Verification items for the finished model (mm, model axes). A direction names the side the tool comes from. Coordinates: 2 decimals unless noted, no trailing zeros. Loops run counter-clockwise (first coordinate to the right, second up) from the corner with the lowest first, then second, coordinate; pieces in that order, holes last. Notation, with made-up numbers: M 30.25,1 L 89.25,1 A24 cw 89.25,36 Z; hole C 73.5,68 d2. An arc over 180 degrees is marked long. Write item = value, one per line. Start each with the question number.
```python
from build123d import *

# Parameters (mm, degrees)
SKETCH_1_W          = 100
SKETCH_1_H          = 100
EXTRUDE_1_DEPTH     = 100
SKETCH_2_W          = 90
SKETCH_2_H          = 75
CUT_EXTRUDE_1_DEPTH = 151
CUT_EXTRUDE_2_REACH = 124.474
SKETCH_3_R          = 7.5
CUT_EXTRUDE_3_REACH = 112.567
SKETCH_4_R          = 1.5
CUT_EXTRUDE_4_DEPTH = 5
SKETCH_6_R          = 1.5
CUT_EXTRUDE_5_DEPTH = 5


with BuildPart() as part:
    # 草圖1 → 填料-伸長1 (new body)
    with BuildSketch(Plane.XY):
        Rectangle(SKETCH_1_W, SKETCH_1_H)
    extrude(amount=EXTRUDE_1_DEPTH)

    # 草圖2 → 除料-伸長1 (cut, through all)
    with BuildSketch(Plane.XZ.offset(50)):
        with Locations((0, 47.5)):
            Rectangle(SKETCH_2_W, SKETCH_2_H)
    extrude(amount=-CUT_EXTRUDE_1_DEPTH, mode=Mode.SUBTRACT)

    # 草圖3 → 除料-伸長2 (cut, up to next)
    with BuildSketch(Plane(origin=(0, 0, 0), x_dir=(-1, 0, 0), z_dir=(0, 0, -1)), mode=Mode.PRIVATE) as cut_extrude_2_sk1:
        Circle(SKETCH_3_R)
    cut_extrude_2_tool1 = extrude(cut_extrude_2_sk1.sketch, amount=-CUT_EXTRUDE_2_REACH, mode=Mode.PRIVATE) & part.part
    add(cut_extrude_2_tool1.solids().sort_by_distance((0, 0, 0))[0], mode=Mode.SUBTRACT)

    # 草圖4 → 除料-伸長3 (cut, up to next)
    with BuildSketch(Plane(origin=(0, 0, 85), x_dir=(-1, 0, 0), z_dir=(0, 0, -1)), mode=Mode.PRIVATE) as cut_extrude_3_sk1:
        with Locations((-32.4, 11.9)):
            Circle(SKETCH_4_R)
    cut_extrude_3_tool1 = extrude(cut_extrude_3_sk1.sketch, amount=-CUT_EXTRUDE_3_REACH, mode=Mode.PRIVATE) & part.part
    # 草圖4 → 除料-伸長3 (cut, up to next)
    with BuildSketch(Plane(origin=(0, 0, 85), x_dir=(-1, 0, 0), z_dir=(0, 0, -1)), mode=Mode.PRIVATE) as cut_extrude_3_sk2:
        with Locations(Location((32.4, 11.9, 0), (0, 0, 180))):
            Circle(SKETCH_4_R)
    cut_extrude_3_tool2 = extrude(cut_extrude_3_sk2.sketch, amount=-CUT_EXTRUDE_3_REACH, mode=Mode.PRIVATE) & part.part
    # 草圖4 → 除料-伸長3 (cut, up to next)
    with BuildSketch(Plane(origin=(0, 0, 85), x_dir=(-1, 0, 0), z_dir=(0, 0, -1)), mode=Mode.PRIVATE) as cut_extrude_3_sk3:
        with Locations((32.4, -11.9)):
            Circle(SKETCH_4_R)
    cut_extrude_3_tool3 = extrude(cut_extrude_3_sk3.sketch, amount=-CUT_EXTRUDE_3_REACH, mode=Mode.PRIVATE) & part.part
    # 草圖4 → 除料-伸長3 (cut, up to next)
    with BuildSketch(Plane(origin=(0, 0, 85), x_dir=(-1, 0, 0), z_dir=(0, 0, -1)), mode=Mode.PRIVATE) as cut_extrude_3_sk4:
        with Locations(Location((-32.4, -11.9, 0), (0, 0, 180))):
            Circle(SKETCH_4_R)
    cut_extrude_3_tool4 = extrude(cut_extrude_3_sk4.sketch, amount=-CUT_EXTRUDE_3_REACH, mode=Mode.PRIVATE) & part.part
    # 草圖4 → 除料-伸長3 (cut, up to next)
    with BuildSketch(Plane(origin=(0, 0, 85), x_dir=(-1, 0, 0), z_dir=(0, 0, -1)), mode=Mode.PRIVATE) as cut_extrude_3_sk5:
        with BuildLine():
            Line((24.9, 24.4), (-24.9, 24.4))
            ThreePointArc((-24.9, 24.4), (-26.314213562, 23.814213562), (-26.9, 22.4))
            Line((-26.9, 22.4), (-26.9, -22.4))
            ThreePointArc((-26.9, -22.4), (-26.314213562, -23.814213562), (-24.9, -24.4))
            Line((-24.9, -24.4), (24.9, -24.4))
            ThreePointArc((24.9, -24.4), (26.314213562, -23.814213562), (26.9, -22.4))
            Line((26.9, -22.4), (26.9, 22.4))
            ThreePointArc((26.9, 22.4), (26.314213562, 23.814213562), (24.9, 24.4))
        make_face()
    cut_extrude_3_tool5 = extrude(cut_extrude_3_sk5.sketch, amount=-CUT_EXTRUDE_3_REACH, mode=Mode.PRIVATE) & part.part
    add(cut_extrude_3_tool1.solids().sort_by_distance((32.4, 11.9, 85))[0], mode=Mode.SUBTRACT)
    add(cut_extrude_3_tool2.solids().sort_by_distance((-32.4, 11.9, 85))[0], mode=Mode.SUBTRACT)
    add(cut_extrude_3_tool3.solids().sort_by_distance((-32.4, -11.9, 85))[0], mode=Mode.SUBTRACT)
    add(cut_extrude_3_tool4.solids().sort_by_distance((32.4, -11.9, 85))[0], mode=Mode.SUBTRACT)
    add(cut_extrude_3_tool5.solids().sort_by_distance((0, 0, 85))[0], mode=Mode.SUBTRACT)

    # 草圖5 → 除料-伸長4 (cut)
    with BuildSketch(Plane.XY.offset(100)):
        with BuildLine():
            Line((-35, 30), (35, 30))
            ThreePointArc((35, 30), (38.535533906, 28.535533906), (40, 25))
            Line((40, 25), (40, -25))
            ThreePointArc((40, -25), (38.535533906, -28.535533906), (35, -30))
            Line((35, -30), (-35, -30))
            ThreePointArc((-35, -30), (-38.535533906, -28.535533906), (-40, -25))
            Line((-40, -25), (-40, 25))
            ThreePointArc((-40, 25), (-38.535533906, 28.535533906), (-35, 30))
        make_face()
    extrude(amount=-CUT_EXTRUDE_4_DEPTH, mode=Mode.SUBTRACT)

    # 草圖6 → 除料-伸長5 (cut)
    # profile 1 of 18: a face of its own
    with BuildSketch(Plane(origin=(0, 0, 85), x_dir=(-1, 0, 0), z_dir=(0, 0, -1))):
        with BuildLine():
            ThreePointArc((-29.239866432, 21), (-32.239866432, 24), (-35.239866432, 21))
            Line((-35.239866432, 21), (-29.239866432, 21))
        make_face()
    # profile 2 of 18: a face of its own
    with BuildSketch(Plane(origin=(0, 0, 85), x_dir=(-1, 0, 0), z_dir=(0, 0, -1))):
        with BuildLine():
            Line((-29.239866432, 21), (-35.239866432, 21))
            ThreePointArc((-35.239866432, 21), (-32.239866432, 18), (-29.239866432, 21))
        make_face()
    # profile 3 of 18: a face of its own
    with BuildSketch(Plane(origin=(0, 0, 85), x_dir=(-1, 0, 0), z_dir=(0, 0, -1))):
        with BuildLine():
            ThreePointArc((-29.239866432, 21), (-32.239866432, 24), (-35.239866432, 21))
            Line((-35.239866432, 21), (-29.239866432, 21))
        make_face()
    # profile 4 of 18: a face of its own
    with BuildSketch(Plane(origin=(0, 0, 85), x_dir=(-1, 0, 0), z_dir=(0, 0, -1))):
        with BuildLine():
            Line((-29.239866432, 21), (-35.239866432, 21))
            ThreePointArc((-35.239866432, 21), (-32.239866432, 18), (-29.239866432, 21))
        make_face()
    # profile 5 of 18: a face of its own
    with BuildSketch(Plane(origin=(0, 0, 85), x_dir=(-1, 0, 0), z_dir=(0, 0, -1))):
        with BuildLine():
            ThreePointArc((-29.239866432, 21), (-32.239866432, 18), (-35.239866432, 21))
            Line((-35.239866432, 21), (-35.239866432, -21))
            ThreePointArc((-35.239866432, -21), (-32.239866432, -18), (-29.239866432, -21))
            Line((-29.239866432, -21), (-29.239866432, 21))
        make_face()
        with Locations((-32.4, -11.9)):
            Circle(SKETCH_6_R, mode=Mode.SUBTRACT)
        with Locations((-32.4, 11.9)):
            Circle(SKETCH_6_R, mode=Mode.SUBTRACT)
    # profile 6 of 18: a face of its own
    with BuildSketch(Plane(origin=(0, 0, 85), x_dir=(-1, 0, 0), z_dir=(0, 0, -1))):
        with BuildLine():
            ThreePointArc((-29.239866432, -21), (-32.239866432, -18), (-35.239866432, -21))
            Line((-35.239866432, -21), (-29.239866432, -21))
        make_face()
    # profile 7 of 18: a face of its own
    with BuildSketch(Plane(origin=(0, 0, 85), x_dir=(-1, 0, 0), z_dir=(0, 0, -1))):
        with BuildLine():
            Line((-29.239866432, -21), (-35.239866432, -21))
            ThreePointArc((-35.239866432, -21), (-32.239866432, -24), (-29.239866432, -21))
        make_face()
    # profile 8 of 18: a face of its own
    with BuildSketch(Plane(origin=(0, 0, 85), x_dir=(-1, 0, 0), z_dir=(0, 0, -1))):
        with BuildLine():
            ThreePointArc((-29.239866432, -21), (-32.239866432, -18), (-35.239866432, -21))
            Line((-35.239866432, -21), (-29.239866432, -21))
        make_face()
    # profile 9 of 18: a face of its own
    with BuildSketch(Plane(origin=(0, 0, 85), x_dir=(-1, 0, 0), z_dir=(0, 0, -1))):
        with BuildLine():
            Line((-29.239866432, -21), (-35.239866432, -21))
            ThreePointArc((-35.239866432, -21), (-32.239866432, -24), (-29.239866432, -21))
        make_face()
    # profile 10 of 18: a face of its own
    with BuildSketch(Plane(origin=(0, 0, 85), x_dir=(-1, 0, 0), z_dir=(0, 0, -1))):
        with BuildLine():
            ThreePointArc((29.239866432, 21), (32.239866432, 18), (35.239866432, 21))
            Line((35.239866432, 21), (29.239866432, 21))
        make_face()
    # profile 11 of 18: a face of its own
    with BuildSketch(Plane(origin=(0, 0, 85), x_dir=(-1, 0, 0), z_dir=(0, 0, -1))):
        with BuildLine():
            Line((29.239866432, 21), (35.239866432, 21))
            ThreePointArc((35.239866432, 21), (32.239866432, 24), (29.239866432, 21))
        make_face()
    # profile 12 of 18: a face of its own
    with BuildSketch(Plane(origin=(0, 0, 85), x_dir=(-1, 0, 0), z_dir=(0, 0, -1))):
        with BuildLine():
            ThreePointArc((29.239866432, 21), (32.239866432, 18), (35.239866432, 21))
            Line((35.239866432, 21), (29.239866432, 21))
        make_face()
    # profile 13 of 18: a face of its own
    with BuildSketch(Plane(origin=(0, 0, 85), x_dir=(-1, 0, 0), z_dir=(0, 0, -1))):
        with BuildLine():
            Line((29.239866432, 21), (35.239866432, 21))
            ThreePointArc((35.239866432, 21), (32.239866432, 24), (29.239866432, 21))
        make_face()
    # profile 14 of 18: a face of its own
    with BuildSketch(Plane(origin=(0, 0, 85), x_dir=(-1, 0, 0), z_dir=(0, 0, -1))):
        with BuildLine():
            ThreePointArc((29.239866432, -21), (32.239866432, -18), (35.239866432, -21))
            Line((35.239866432, -21), (35.239866432, 21))
            ThreePointArc((35.239866432, 21), (32.239866432, 18), (29.239866432, 21))
            Line((29.239866432, 21), (29.239866432, -21))
        make_face()
        with Locations((32.4, -11.9)):
            Circle(SKETCH_6_R, mode=Mode.SUBTRACT)
        with Locations((32.4, 11.9)):
            Circle(SKETCH_6_R, mode=Mode.SUBTRACT)
    # profile 15 of 18: a face of its own
    with BuildSketch(Plane(origin=(0, 0, 85), x_dir=(-1, 0, 0), z_dir=(0, 0, -1))):
        with BuildLine():
            ThreePointArc((29.239866432, -21), (32.239866432, -24), (35.239866432, -21))
            Line((35.239866432, -21), (29.239866432, -21))
        make_face()
    # profile 16 of 18: a face of its own
    with BuildSketch(Plane(origin=(0, 0, 85), x_dir=(-1, 0, 0), z_dir=(0, 0, -1))):
        with BuildLine():
            Line((29.239866432, -21), (35.239866432, -21))
            ThreePointArc((35.239866432, -21), (32.239866432, -18), (29.239866432, -21))
        make_face()
    # profile 17 of 18: a face of its own
    with BuildSketch(Plane(origin=(0, 0, 85), x_dir=(-1, 0, 0), z_dir=(0, 0, -1))):
        with BuildLine():
            ThreePointArc((29.239866432, -21), (32.239866432, -24), (35.239866432, -21))
            Line((35.239866432, -21), (29.239866432, -21))
        make_face()
    # profile 18 of 18: a face of its own
    with BuildSketch(Plane(origin=(0, 0, 85), x_dir=(-1, 0, 0), z_dir=(0, 0, -1))):
        with BuildLine():
            Line((29.239866432, -21), (35.239866432, -21))
            ThreePointArc((35.239866432, -21), (32.239866432, -18), (29.239866432, -21))
        make_face()
    extrude(amount=-CUT_EXTRUDE_5_DEPTH, mode=Mode.SUBTRACT)


solid = part.part
```
Q1. Gauge pin test, flat end, axial feed: pin 1 (2.5 mm diameter, centred on x = -32.4, y = 11.9, fed in from +Z). Record the tip position at first contact, or that the pin passes through.
Q2. Sectioned sample at D-D on x = 18.5. Record the cut outline in (y, z), plus the area to 3 significant figures.
Q3. Mould release check, pull along Z, two halves, no side actions. Record for faces 1 (the face through (33.83, -12.35, 92.46)), 2 (the face through (27.2, 0.4, 95)), 3 (the face through (35.24, 0, 87)): +Z half, -Z half, draft (parallel to the pull), parting line (faces both ways), or undercut.
Q4. Sectioned sample at C-C on y = 11.9. Count the separate pieces of the cut face and the enclosed holes in it, plus the area to 3 significant figures.
Q5. Scan lines: L1, parallel to Y at x = 12.5, z = 93.5; L2, parallel to Z at x = 29, y = 13.5; L3, parallel to X at y = -45, z = 36.5. Record each from-to range of solid material in increasing order. Write a range as [from, to].
Q6. Sectioned sample at A-A on x = -38. Record the cut outline in (y, z).
Q7. Sectioned sample at B-B on z = 80. Record the cut outline in (x, y), plus the area to 3 significant figures.
Q8. Set-up check for faces 4 (the face through (-40, 0, 98)), 5 (the face through (-45, -1, 47)), 6 (the face through (-32.2, -24, 87.5)): record each of +Z, -Z, +X, -X, +Y, -Y from which the full face is reachable in a straight line by a thin tool's end or side.
Solutions:
q1.pin_1 = 10
q2.outline = M -50,0 L 50,0 L 50,10 L -50,10 Z; M -50,85 L -24.4,85 L -24.4,95 L -30,95 L -30,100 L -50,100 Z; M 24.4,85 L 50,85 L 50,100 L 30,100 L 30,95 L 24.4,95 Z
q2.area = 1,710 mm²
q3.face_1 = draft
q3.face_2 = +Z half
q3.face_3 = undercut
q4.separate_pieces = 3
q4.enclosed_holes = 0
q4.area = 2,220 mm²
q5.L1 = [-50, -24.4], [24.4, 50]
q5.L2 = [0, 10], [85, 95]
q5.L3 = [-50, -45], [45, 50]
q6.outline = M -50,0 L 50,0 L 50,10 L -50,10 Z; M -50,85 L 50,85 L 50,100 L 29,100 L 29,95 L -29,95 L -29,100 L -50,100 Z
q7.outline = M -50,-50 L -45,-50 L -45,50 L -50,50 Z; M 45,-50 L 50,-50 L 50,50 L 45,50 Z
q7.area = 1,000 mm²
q8.face_4 = +Z
q8.face_5 = +Y, -Y
q8.face_6 = none
